```python
from build123d import *

# Parameters (mm, degrees)
SKETCH1_W               = 60
SKETCH1_H               = 60
BOSS_EXTRUDE1_DEPTH     = 100
SKETCH2_W               = 10.95
SKETCH2_H               = 10.95
CUT_EXTRUDE1_DEPTH      = 93
MIRROR2_COPY_1_SKETCH_W = 10.95
MIRROR2_COPY_1_SKETCH_H = 10.95
MIRROR2_COPY_1_DEPTH    = 93
SKETCH5_R               = 2.5
CUT_EXTRUDE2_DEPTH      = 93
SKETCH7_R               = 19.05
BOSS_EXTRUDE4_DEPTH     = 1.8
SKETCH8_R               = 4
BOSS_EXTRUDE5_DEPTH     = 20.4
FILLET2_R               = 5
SKETCH15_R              = 4
BOSS_EXTRUDE6_DEPTH     = 13.6
FILLET4_R               = 1
CUT_EXTRUDE4_DEPTH      = 15.5
BOSS_EXTRUDE7_DEPTH     = 9
BOSS_EXTRUDE8_DEPTH     = 9
SKETCH22_R              = 1.25
SKETCH22_R_2            = 2
CUT_EXTRUDE7_DEPTH      = 4


with BuildPart() as part:
    # Sketch1 → Boss-Extrude1 (new body)
    with BuildSketch(Plane(origin=(0, 0, 0), x_dir=(1, 0, 0), z_dir=(0, 1, 0))):
        Rectangle(SKETCH1_W, SKETCH1_H)
    extrude(amount=BOSS_EXTRUDE1_DEPTH)

    # Sketch2 → Cut-Extrude1 (cut)
    with BuildSketch(Plane(origin=(0, 100, 0), x_dir=(1, 0, 0), z_dir=(0, 1, 0))):
        with Locations((-24.525, 24.525)):
            Rectangle(SKETCH2_W, SKETCH2_H)
    cut_extrude1 = extrude(amount=-CUT_EXTRUDE1_DEPTH, mode=Mode.SUBTRACT)

    # Mirror1: Cut-Extrude1 across plane
    add(cut_extrude1.mirror(Plane(origin=(0, 0, 0), x_dir=(0, 0, 1), z_dir=(1, 0, 0))), mode=Mode.SUBTRACT)

    # Mirror2: Cut-Extrude1 across plane
    add(cut_extrude1.mirror(Plane.XY), mode=Mode.SUBTRACT)

    # Mirror2 copy 1 sketch → Mirror2 copy 1 (cut)
    with BuildSketch(Plane(origin=(0, 100, 0), x_dir=(-1, 0, 0), z_dir=(0, 1, 0))):
        with Locations((-24.525, 24.525)):
            Rectangle(MIRROR2_COPY_1_SKETCH_W, MIRROR2_COPY_1_SKETCH_H)
    extrude(amount=-MIRROR2_COPY_1_DEPTH, mode=Mode.SUBTRACT)

    # Sketch5 → Cut-Extrude2 (cut)
    with BuildSketch(Plane.XZ):
        with Locations((-23.57, -23.57)):
            Circle(SKETCH5_R)
        with Locations((23.57, -23.57)):
            Circle(SKETCH5_R)
        with Locations((23.57, 23.57)):
            Circle(SKETCH5_R)
        with Locations((-23.57, 23.57)):
            Circle(SKETCH5_R)
    extrude(amount=-CUT_EXTRUDE2_DEPTH, mode=Mode.SUBTRACT)

    # Sketch7 → Boss-Extrude4 (add)
    with BuildSketch(Plane.XZ):
        Circle(SKETCH7_R)
    extrude(amount=BOSS_EXTRUDE4_DEPTH)

    # Sketch8 → Boss-Extrude5 (add)
    with BuildSketch(Plane.XZ.offset(1.8)):
        Circle(SKETCH8_R)
    extrude(amount=BOSS_EXTRUDE5_DEPTH)

    # Fillet2
    fillet2_edges = [part.edges().sort_by_distance(p)[0] for p in [
        (-30, 3.5, -30),
        (30, 3.5, -30),
        (30, 3.5, 30),
        (-30, 3.5, 30),
    ]]
    fillet(fillet2_edges, radius=FILLET2_R)

    # Sketch15 → Boss-Extrude6 (add)
    with BuildSketch(Plane(origin=(0, 100, 0), x_dir=(1, 0, 0), z_dir=(0, 1, 0))):
        Circle(SKETCH15_R)
    extrude(amount=BOSS_EXTRUDE6_DEPTH)

    # Fillet4
    fillet4_edges = [part.edges().sort_by_distance(p)[0] for p in [
        (-4, 113.6, 0),
    ]]
    fillet(fillet4_edges, radius=FILLET4_R)

    # Sketch17 → Cut-Extrude4 (cut)
    with BuildSketch(Plane.XZ.offset(22.2)):
        with BuildLine():
            Line((-2.552821159, -3.1), (2.552821159, -3.1))
            ThreePointArc((2.552821159, -3.1), (0, -4.015830658), (-2.552821159, -3.1))
        make_face()
    extrude(amount=-CUT_EXTRUDE4_DEPTH, mode=Mode.SUBTRACT)

    # Sketch20 → Boss-Extrude7 (add)
    with BuildSketch(Plane(origin=(0, 0, -30), x_dir=(-1, 0, 0), z_dir=(0, 0, -1))):
        Polygon((0, 100), (10.5, 100), (10.5, 83), (-10.5, 83), (-10.5, 100), align=None)
    extrude(amount=BOSS_EXTRUDE7_DEPTH)

    # Sketch21 → Boss-Extrude8 (add)
    with BuildSketch(Plane.XZ.offset(-83)):
        Polygon((0, -39), (-6, -39), (-6, -34), (6, -34), (6, -39), align=None)
    extrude(amount=BOSS_EXTRUDE8_DEPTH)

    # Sketch22 → Cut-Extrude7 (cut)
    with BuildSketch(Plane(origin=(0, 100, 0), x_dir=(1, 0, 0), z_dir=(0, 1, 0))):
        with Locations((-9.575, 0)):
            Circle(SKETCH22_R)
        with Locations((9.575, 0)):
            Circle(SKETCH22_R)
        with Locations((-8.20848344, 22.552622899)):
            Circle(SKETCH22_R_2)
        with Locations((-15.426902632, -18.385066635)):
            Circle(SKETCH22_R_2)
        with Locations((23.635386072, -4.167556264)):
            Circle(SKETCH22_R_2)
    extrude(amount=-CUT_EXTRUDE7_DEPTH, mode=Mode.SUBTRACT)


solid = part.part
```
Design review of the part built by this model. Coordinates are the model's own, in mm. A direction names the side the tool comes from. Round coordinates to 2 decimals unless told otherwise and drop trailing zeros. Order: outer loops, then holes, each group sorted by start corner. A loop starts at its lowest first (then second) coordinate and runs counter-clockwise, first axis right, second up. Notation, with made-up numbers: M 87,-21 L 126,-21 A20 cw 126,10 Z; hole C -5.75,-25 d5. An arc over 180 degrees is marked long. Put each result on its own line as item: value.
Q1. Consider section B-B (z = 23.57). State the section outline as (x, y) points, and give its area (3 significant figures).
Reported:
outline: M -30,0 L -26.07,0 L -26.07,7 L -30,7 Z; M -21.07,0 L 21.07,0 L 21.07,7 L 19.05,7 L 19.05,100 L -19.05,100 L -19.05,7 L -21.07,7 Z; M 26.07,0 L 30,0 L 30,7 L 26.07,7 Z
area: 3,890 mm²
Q2. To check wall thickness, follow line 1 (X direction, y = 98.7, z = 0) (3 decimals); line 2 (Y direction, x = -13.5, z = 9); line 3 (X direction, y = 53.5, z = 26). State the ranges of each line that lie inside material, in increasing order.
Reported:
line 1: -30 to -10.825, -8.325 to 8.325, 10.825 to 30
line 2: -1.8 to 100
line 3: -19.05 to 19.05
Q3. Consider section C-C (x = 0). State the section outline as (y, z) points, and give its area (3 significant figures).
Reported:
outline: M -22.2,-3.1 L -6.7,-3.1 L -6.7,-4 L -1.8,-4 L -1.8,-19.05 L 0,-19.05 L 0,-30 L 83,-30 L 83,-34 L 74,-34 L 74,-39 L 100,-39 L 100,-4 L 112.6,-4 A1 ccw 113.6,-3 L 113.6,3 A1 ccw 112.6,4 L 100,4 L 100,30 L 0,30 L 0,19.05 L -1.8,19.05 L -1.8,4 L -22.2,4 Z
area: 6,520 mm²
Q4. Consider section D-D (z = 9). State the section outline as (x, y) points.
Reported:
outline: M -30,0 L -16.79,0 L -16.79,-1.8 L 16.79,-1.8 L 16.79,0 L 30,0 L 30,100 L -30,100 Z
Q5. Consider section A-A (y = 78). State the section outline as (x, z) points.
Reported:
outline: M -30,-19.05 L -19.05,-19.05 L -19.05,-30 L 19.05,-30 L 19.05,-19.05 L 30,-19.05 L 30,19.05 L 19.05,19.05 L 19.05,30 L -19.05,30 L -19.05,19.05 L -30,19.05 Z; M -6,-39 L 6,-39 L 6,-34 L -6,-34 Z
Q6. Insertion check: pin 1 Ø2.5 at (x, z) = (-1, -37.5) entering from -Y; pin 2 Ø1.5 at (x, z) = (-2, 4.5) entering from -Y; pin 3 Ø3.5 at (x, z) = (25, 23.5) entering from +Y. Each pin has a flat end and moves straight along its axis. Give the tip position at first contact, or say it passes through.
Reported:
pin 1: y = 74
pin 2: y = -1.8
pin 3: y = 7
Q7. Draft analysis for pull direction Z (two halves, no side actions). For faces 4 (the face through (-8, 96, -23)), 5 (the face through (10.5, 91, -34)), 6 (the face through (-15.12, -0.89, -11.59)), state which applies: released by +Z, released by -Z, zero draft, split by the parting line, or undercut.
Reported:
face 4: undercut
face 5: zero draft
face 6: split by the parting line
Q8. Machinability: for faces 1 (the face through (6, 79, -36)), 2 (the face through (-19.05, 54, 24)), 3 (the face through (-10, 96, 0)), which of the approach directions +Z, -Z, +X, -X, +Y, -Y give a long, thin tool a straight path to every point of the face, cutting with its end or side? Answer none if there is none.
Reported:
face 1: -Z, +X, -Y
face 2: +Z, -X, +Y
face 3: +Y
